from build123d import *

# Parameters (mm, degrees)
BOSS_EXTRUDE1_DEPTH     = 12
SKETCH1_3_R             = 1
SKETCH1_3_R_2           = 5
CUT_EXTRUDE1_DEPTH      = 3
SKETCH1_4_R             = 1
SKETCH1_4_R_2           = 5
CUT_EXTRUDE2_DEPTH      = 13
BOSS_EXTRUDE2_DEPTH     = 8
BOSS_EXTRUDE3_DEPTH     = 10
CUT_EXTRUDE5_DEPTH      = 8
SKETCH3_7_R             = 10
CUT_EXTRUDE6_DEPTH      = 46
SKETCH7_R               = 1.280379455
CUT_EXTRUDE7_DEPTH      = 3
SKETCH9_R               = 1.5
CUT_EXTRUDE8_DEPTH      = 38
CUT_EXTRUDE8_DEPTH_BACK = 9


with BuildPart() as part:
    # Sketch1 → Boss-Extrude1 (new body)
    with BuildSketch(Plane.XY):
        with BuildLine():
            Line((0, 45), (0, 10))
            ThreePointArc((0, 10), (2.928932188, 2.928932188), (10, 0))
            Line((10, 0), (35, 0))
            ThreePointArc((35, 0), (42.071067812, 2.928932188), (45, 10))
            Line((45, 10), (45, 25.947441117))
            ThreePointArc((45, 25.947441117), (43.660254038, 30.947441117), (40, 34.607695155))
            Line((40, 34.607695155), (22, 45))
            Line((22, 45), (0, 45))
        make_face()
    extrude(amount=-BOSS_EXTRUDE1_DEPTH)

    # Sketch1<3> → Cut-Extrude1 (cut)
    with BuildSketch(Plane.XY):
        with Locations((22, 25)):
            Circle(SKETCH1_3_R)
        with BuildLine():
            ThreePointArc((16, 26), (16.585786438, 27.414213562), (18, 28))
            Line((18, 28), (26, 28))
            ThreePointArc((26, 28), (27.414213562, 27.414213562), (28, 26))
            Line((28, 26), (28, 10))
            ThreePointArc((28, 10), (27.414213562, 8.585786438), (26, 8))
            Line((26, 8), (18, 8))
            ThreePointArc((18, 8), (16.585786438, 8.585786438), (16, 10))
            Line((16, 10), (16, 26))
        make_face()
        with Locations((22, 25)):
            Circle(SKETCH1_3_R, mode=Mode.SUBTRACT)
        with Locations((22, 11)):
            Circle(SKETCH1_3_R, mode=Mode.SUBTRACT)
        with Locations((22, 11)):
            Circle(SKETCH1_3_R)
        with Locations((22, 18)):
            Circle(SKETCH1_3_R_2)
    extrude(amount=-CUT_EXTRUDE1_DEPTH, mode=Mode.SUBTRACT)

    # Sketch1<4> → Cut-Extrude2 (cut, through all)
    with BuildSketch(Plane.XY):
        with Locations((22, 25)):
            Circle(SKETCH1_4_R)
        with Locations((22, 11)):
            Circle(SKETCH1_4_R)
        with Locations((22, 18)):
            Circle(SKETCH1_4_R_2)
    extrude(amount=-CUT_EXTRUDE2_DEPTH, mode=Mode.SUBTRACT)

    # Sketch3 → Boss-Extrude2 (add)
    with BuildSketch(Plane.ZY):
        with BuildLine():
            Line((0, 45), (9.192533317, 52.713451316))
            Line((9.192533317, 52.713451316), (9.192533317, 83.893517708))
            Line((9.192533317, 83.893517708), (1.915111108, 90))
            Line((1.915111108, 90), (-28.48263132, 90))
            ThreePointArc((-28.48263132, 90), (-30.595722628, 89.531538935), (-32.312853535, 88.213938048))
            Line((-32.312853535, 88.213938048), (-35.850897987, 83.997460862))
            Line((-35.850897987, 83.997460862), (-39.307466683, 83.997460862))
            ThreePointArc((-39.307466683, 83.997460862), (-44.964320932, 81.654315111), (-47.307466683, 75.997460862))
            Line((-47.307466683, 75.997460862), (-47.307466683, 58))
            ThreePointArc((-47.307466683, 58), (-44.964320932, 52.343145751), (-39.307466683, 50))
            Line((-39.307466683, 50), (-35.850897987, 50))
            Line((-35.850897987, 50), (-34.340222638, 47.408116517))
            ThreePointArc((-34.340222638, 47.408116517), (-32.502582275, 45.585533814), (-29.999847687, 44.925951074))
            Line((-29.999847687, 44.925951074), (-12, 45))
            Line((-12, 45), (0, 45))
        make_face()
        with BuildLine():
            ThreePointArc((-0.307466683, 58), (-0.89325312, 56.585786438), (-2.307466683, 56))
            Line((-2.307466683, 56), (-39.307466683, 56))
            ThreePointArc((-39.307466683, 56), (-40.721680245, 56.585786438), (-41.307466683, 58))
            Line((-41.307466683, 58), (-41.307466683, 76))
            ThreePointArc((-41.307466683, 76), (-40.721680245, 77.414213562), (-39.307466683, 78))
            Line((-39.307466683, 78), (-2.307466683, 78))
            ThreePointArc((-2.307466683, 78), (-0.89325312, 77.414213562), (-0.307466683, 76))
            Line((-0.307466683, 76), (-0.307466683, 58))
        make_face(mode=Mode.SUBTRACT)
    extrude(amount=-BOSS_EXTRUDE2_DEPTH)

    # Sketch3<4> → Boss-Extrude3 (add)
    with BuildSketch(Plane.ZY):
        with BuildLine():
            Line((-43.307466683, 75.997460862), (-43.307466683, 58))
            ThreePointArc((-43.307466683, 58), (-42.135893807, 55.171572875), (-39.307466683, 54))
            Line((-39.307466683, 54), (-2.307466683, 54))
            ThreePointArc((-2.307466683, 54), (0.520960442, 55.171572875), (1.692533317, 58))
            Line((1.692533317, 58), (1.692533317, 75.997460862))
            ThreePointArc((1.692533317, 75.997460862), (0.520960442, 78.825887987), (-2.307466683, 79.997460862))
            Line((-2.307466683, 79.997460862), (-39.307466683, 79.997460862))
            ThreePointArc((-39.307466683, 79.997460862), (-42.135893807, 78.825887987), (-43.307466683, 75.997460862))
        make_face()
    extrude(amount=-BOSS_EXTRUDE3_DEPTH)

    # Sketch3<6> → Cut-Extrude5 (cut)
    with BuildSketch(Plane.ZY):
        with BuildLine():
            Line((-41.307466683, 76), (-41.307466683, 58))
            ThreePointArc((-41.307466683, 58), (-40.721680245, 56.585786438), (-39.307466683, 56))
            Line((-39.307466683, 56), (-2.307466683, 56))
            ThreePointArc((-2.307466683, 56), (-0.89325312, 56.585786438), (-0.307466683, 58))
            Line((-0.307466683, 58), (-0.307466683, 76))
            ThreePointArc((-0.307466683, 76), (-0.89325312, 77.414213562), (-2.307466683, 78))
            Line((-2.307466683, 78), (-39.307466683, 78))
            ThreePointArc((-39.307466683, 78), (-40.721680245, 77.414213562), (-41.307466683, 76))
        make_face()
    extrude(amount=-CUT_EXTRUDE5_DEPTH, mode=Mode.SUBTRACT)

    # Sketch3<7> → Cut-Extrude6 (cut, through all)
    with BuildSketch(Plane.ZY):
        with Locations((-11.307466683, 67)):
            Circle(SKETCH3_7_R)
    extrude(amount=-CUT_EXTRUDE6_DEPTH, mode=Mode.SUBTRACT)

    # Sketch7 → Cut-Extrude7 (cut)
    with BuildSketch(Plane.ZY):
        with Locations((-44.307466683, 72)):
            Circle(SKETCH7_R)
        with Locations((-44.307466683, 62)):
            Circle(SKETCH7_R)
        with Locations((2.692533317, 62)):
            Circle(SKETCH7_R)
        with Locations((2.692533317, 72)):
            Circle(SKETCH7_R)
    extrude(amount=-CUT_EXTRUDE7_DEPTH, mode=Mode.SUBTRACT)

    # Sketch9 → Cut-Extrude8 (cut, two sides)
    with BuildSketch(Plane(origin=(8, 0, 0), x_dir=(0, 0, -1), z_dir=(1, 0, 0))) as cut_extrude8_sk:
        with Locations((3.333760106, 85.147460862)):
            Circle(SKETCH9_R)
        with Locations((23.283760106, 85.147460862)):
            Circle(SKETCH9_R)
    extrude(amount=CUT_EXTRUDE8_DEPTH, mode=Mode.SUBTRACT)
    extrude(cut_extrude8_sk.sketch, amount=-CUT_EXTRUDE8_DEPTH_BACK, mode=Mode.SUBTRACT)


solid = part.part
CAD build for the part. Positions are in the model's coordinates, mm. A direction names the side the tool comes from. Give positions to 0.01 mm unless a question says otherwise; leave off trailing zeros. Write each loop counter-clockwise with the first axis right and the second up, starting at its lowest first coordinate (ties: lowest second). Pieces come first, ordered by that corner, then holes. Notation, with made-up numbers: (30.5, 72) - (68.5, 72) arc R20 cw to (68.5, 109) - close; hole circle Ø3 at (5, 4.25). An arc over 180 degrees is marked (long way). Put each result on its own line as item: value.
(1) Saw through at D-D (x = 41). List the corners of the cut face in (y, z), then the cut area to 3 significant figures.
Working result:
outline: (2, -12) - (33.95, -12) - (33.95, 0) - (2, 0) - close
area: 383 mm^2
(2) Saw through at A-A (y = 67). List the corners of the cut face in (x, z), then the cut area to 3 significant figures.
Working result:
outline: (0, -47.31) - (8, -47.31) - (8, -43.31) - (10, -43.31) - (10, -21.31) - (8, -21.31) - (8, -41.31) - (0, -41.31) - close; (0, -0.31) - (8, -0.31) - (8, -1.31) - (10, -1.31) - (10, 1.69) - (8, 1.69) - (8, 9.19) - (0, 9.19) - close
area: 174 mm^2
(3) Drop flat-ended pins along their axis: pin 1 Ø3.5 at (x, z) = (22.5, -1.5) entering from +Y; pin 2 Ø5 at (x, z) = (40.5, 1) entering from -Y; pin 3 Ø2 at (y, z) = (72, 2.69) entering from -X. Give the stop position or say it passes through.
Working result:
pin 1: y = 45
pin 2: y = 0.53
pin 3: x = 3
(4) Pull direction X, two halves, no side cores. Call faces 6 (the cylindrical face through (16.57, 27.4, -1.48)), 7 (the flat face through (0, 51, -13)), 8 (the cylindrical face through (3.944, 89.544, -30.568)): released by +X, released by -X, zero draft, split by the parting line, or undercut.
Working result:
face 6: undercut
face 7: released by -X
face 8: zero draft
(5) Saw through at B-B (z = -15). List the corners of the cut face in (x, y).
Working result:
outline: (0, 44.99) - (8, 44.99) - (8, 54) - (10, 54) - (10, 57.71) - (8, 57.71) - (8, 56) - (0, 56) - close; (0, 78) - (8, 78) - (8, 76.29) - (10, 76.29) - (10, 80) - (8, 80) - (8, 90) - (0, 90) - close
(6) Tool access for faces 1 (the flat face through (3, 72, 3)), 2 (the flat face through (9, 67, -43.307)), 3 (the cylindrical face through (8.99, 78.86, -42.1)), 4 (the cylindrical face through (8.986, 55.203, -42.167)), 5 (the flat face through (22, 28, -1)): list every direction of +Z, -Z, +X, -X, +Y, -Y with a clear straight run to the whole face (end or side of a thin tool).
Working result:
face 1: -X
face 2: -Z, +X, +Y, -Y
face 3: -Z, +X, +Y
face 4: -Z, +X, -Y
face 5: +Z
(7) Saw through at C-C (y = 79). List the corners of the cut face in (x, z), then the cut area to 3 significant figures.
Working result:
outline: (0, -46.72) - (8, -46.72) - (8, -41.95) - (10, -41.95) - (10, 0.34) - (8, 0.34) - (8, 9.19) - (0, 9.19) - close
area: 532 mm^2
(8) Wall check: L1, parallel to Y at x = 22, z = -6; L2, parallel to Y at x = 2.5, z = -24.5; L3, parallel to Z at x = 39, y = 13. Give the ranges that are in metal, low to high.
Working result:
L1: 0 to 10, 12 to 13, 23 to 24, 26 to 45
L2: 44.95 to 56, 78 to 84.27, 86.03 to 90
L3: -12 to 0
